```python
from build123d import *
from build123d.topology import SkipClean

# Parameters (mm, degrees)
SKETCH_3_W          = 40
SKETCH_3_H          = 40
CUT_EXTRUDE_1_DEPTH = 70
CUT_REVOLVE_1_ANGLE = 90
CUT_EXTRUDE_2_DEPTH = 452.082032598
EXTRUDE_1_DEPTH     = 42
SKETCH_7_R          = 10
CUT_EXTRUDE_3_DEPTH = 440
CUT_EXTRUDE_4_DEPTH = 22
SKETCH_9_W          = 60
SKETCH_9_H          = 30
CUT_EXTRUDE_5_DEPTH = 30


with BuildPart() as part:
    # 草图1 → 旋转3 (revolve)
    with SkipClean():  # the faces are left unmerged after this step: merging them gives an invalid solid
        with BuildSketch(Plane(origin=(0, 0, 0), x_dir=(1, 0, 0), z_dir=(0, 1, 0))):
            with BuildLine():
                add(Edge.make_bspline(
                    [(200, 0), (200, 125), (0, 125), (-200, 125), (-200, 0)],
                    knots=[0, 0, 0, 1.570796327, 1.570796327, 3.141592654, 3.141592654, 3.141592654], degree=2, weights=[1, 0.707106781, 1, 0.707106781, 1]))
                Line((-200, 0), (200, 0))
            make_face()
            with BuildLine():
                Line((200, 0), (-200, 0))
                add(Edge.make_bspline(
                    [(-200, 0), (-200, -125), (0, -125), (200, -125), (200, 0)],
                    knots=[3.141592654, 3.141592654, 3.141592654, 4.71238898, 4.71238898, 6.283185307, 6.283185307, 6.283185307], degree=2, weights=[1, 0.707106781, 1, 0.707106781, 1]))
            make_face()
        revolve(axis=Axis((-376.776806715, 0, 0), (1, 0, 0)))
    add(part.part.scale(1), mode=Mode.REPLACE)  # the faces are merged on a copy

    # Surface Cut 1
    split(bisect_by=Plane.XY, keep=Keep.BOTTOM)

    # 草图3 → 切除-拉伸1 (cut)
    with BuildSketch(Plane(origin=(0, -125.246294878, -45.585923288), x_dir=(1, 0, 0), z_dir=(0, 0.9396926207859081, 0.34202014332566943))):
        with Locations((0, 43.622733675)):
            Rectangle(SKETCH_3_W, SKETCH_3_H)
    extrude(amount=CUT_EXTRUDE_1_DEPTH, mode=Mode.SUBTRACT)

    # 草图4 → 切除-旋转1 (revolve, cut)
    with BuildSketch(Plane.XY):
        with BuildLine():
            Line((-189.264857791, 10), (189.264857791, 10))
            add(Edge.make_bspline(
                [(189.264857791, 10), (189.01661408, 11.685645813), (188.399842232, 15.02459428), (186.660672029, 21.717695752), (183.544014825, 30.028723701), (178.280438028, 39.871100011), (169.238112825, 52.698753606), (154.190025082, 67.938441209), (130.617285564, 84.133702491), (102.331625356, 97.503941795), (70.346299789, 107.469826997), (35.819572857, 113.615740598), (0, 115.692129701), (-35.819572857, 113.615740598), (-70.346299789, 107.469826997), (-102.331625356, 97.503941795), (-130.617285564, 84.133702491), (-154.190025082, 67.938441209), (-169.238112825, 52.698753606), (-178.280438028, 39.871100011), (-183.544014825, 30.028723701), (-186.660672029, 21.717695752), (-188.399842232, 15.02459428), (-189.01661408, 11.685645813), (-189.264857791, 10)],
                knots=[0.091784635, 0.091784635, 0.091784635, 0.091784635, 0.13800375, 0.184222866, 0.276661096, 0.369099327, 0.461537558, 0.646414019, 0.831290481, 1.016166942, 1.201043404, 1.385919865, 1.570796327, 1.755672788, 1.94054925, 2.125425711, 2.310302173, 2.495178634, 2.680055096, 2.772493326, 2.864931557, 2.957369788, 3.003588903, 3.049808019, 3.049808019, 3.049808019, 3.049808019], degree=3))
        make_face()
    revolve(axis=Axis((-200, 0, 0), (-1, 0, 0)), revolution_arc=CUT_REVOLVE_1_ANGLE, mode=Mode.SUBTRACT)

    # 草图5 → 切除-拉伸2 (cut, through all)
    with BuildSketch(Plane(origin=(215, 0, 0), x_dir=(0, 0, -1), z_dir=(1, 0, 0))):
        with BuildLine():
            ThreePointArc((20, 20), (40, 0), (20, -20))
            Line((20, -20), (0, -20))
            Line((0, -20), (0, 20))
            Line((0, 20), (20, 20))
        make_face()
    extrude(amount=-CUT_EXTRUDE_2_DEPTH, mode=Mode.SUBTRACT)

    # 草图6 → 凸台-拉伸1 (add)
    with BuildSketch(Plane(origin=(215, 0, 0), x_dir=(0, 0, -1), z_dir=(1, 0, 0))):
        with BuildLine():
            Line((20, -20), (0, -20))
            Line((0, -20), (0, 20))
            Line((0, 20), (20, 20))
            ThreePointArc((20, 20), (40, 0), (20, -20))
        make_face()
    extrude_1 = extrude(amount=-EXTRUDE_1_DEPTH)

    # 镜向1: 凸台-拉伸1 across plane
    add(extrude_1.mirror(Plane(origin=(0, 0, 0), x_dir=(0, 0, 1), z_dir=(1, 0, 0))))

    # 草图7 → 切除-拉伸3 (cut)
    with BuildSketch(Plane(origin=(215, 0, 0), x_dir=(0, 0, -1), z_dir=(1, 0, 0))):
        with Locations(Location((20, 0, 0), (0, 0, 180))):
            Circle(SKETCH_7_R)
    extrude(amount=-CUT_EXTRUDE_3_DEPTH, mode=Mode.SUBTRACT)

    # 草图8 → 切除-拉伸4 (cut)
    with BuildSketch(Plane(origin=(215, 0, 0), x_dir=(0, 0, -1), z_dir=(1, 0, 0))):
        with BuildLine():
            ThreePointArc((0, 4.7e-08), (5.857864393, 14.14213564), (20, 20))
            Line((20, 20), (0, 20))
            Line((0, 20), (0, 4.7e-08))
        make_face()
        with BuildLine():
            ThreePointArc((20, -20), (5.85786436, -14.142135607), (0, 4.7e-08))
            Line((0, 4.7e-08), (0, -20))
            Line((0, -20), (20, -20))
        make_face()
    cut_extrude_4 = extrude(amount=-CUT_EXTRUDE_4_DEPTH, mode=Mode.SUBTRACT)

    # 镜向2: 切除-拉伸4 across plane
    add(cut_extrude_4.mirror(Plane(origin=(0, 0, 0), x_dir=(0, 0, 1), z_dir=(1, 0, 0))), mode=Mode.SUBTRACT)

    # 草图9 → 切除-拉伸5 (cut)
    with BuildSketch(Plane(origin=(0, -126.642161547, -22.330429976), x_dir=(1, 0, 0), z_dir=(0, 0.984807753012208, 0.17364817766693072))):
        with Locations((0, 13.014685424)):
            Rectangle(SKETCH_9_W, SKETCH_9_H)
    extrude(amount=CUT_EXTRUDE_5_DEPTH, mode=Mode.SUBTRACT)


solid = part.part
```
CAD build for the part. Positions are in the model's coordinates, mm. A direction names the side the tool comes from. Round coordinates to 2 decimals unless told otherwise and drop trailing zeros. Write item = value, one per line. Start each with the question number.
Q1. Drop flat-ended pins along their axis: pin 1 (12 mm diameter, centred on y = 0, z = -20, fed in from -X); pin 2 (6 mm diameter, centred on x = 27, y = -65, fed in from -Z); pin 3 (4 mm diameter, centred on x = 180, z = -8, fed in from +Y); pin 4 (1 mm diameter, centred on x = 95, z = -70, fed in from +Y). Give the stop position or say it passes through.
Q2. Which spindle directions (+Z, -Z, +X, -X, +Y, -Y) get a long thin tool onto all of the face, cutting with end or side? Do faces 4 (the flat face through (-193, -15, -4)), 5 (the flat face through (-173, 0, -7)), 6 (the flat face through (-0.28, -79.718, -54.154)). Say none if no direction does.
Q3. Probe L1, parallel to X at y = -15, z = -13.5; L2, parallel to Y at x = -33, z = -19; L3, parallel to X at y = 28, z = -13. List the from-to ranges inside material, lowest first. Write a range as from..to.
Q4. Mould opens along Y. For faces 1 (the flat face through (-215, 9, -25)), 2 (the flat face through (-0.42, -103.829, -46.755)), 3 (the flat face through (-0.42, -110.62, -17.49)) say: pulls with the +Y half, pulls with the -Y half, needs draft (parallel to the pull), parting line crosses it, or undercut.
Answers below:
q1.pin_1 = through
q1.pin_2 = -107.24
q1.pin_3 = 56.45
q1.pin_4 = 85.31
q2.face_4 = +Z, -X
q2.face_5 = +Z
q2.face_6 = none
q3.L1 = -215..-173, 173..215
q3.L2 = -121.81..-20, 111.62..121.81
q3.L3 = -193.8..-182.89, 182.89..193.8
q4.face_1 = needs draft
q4.face_2 = pulls with the -Y half
q4.face_3 = undercut
